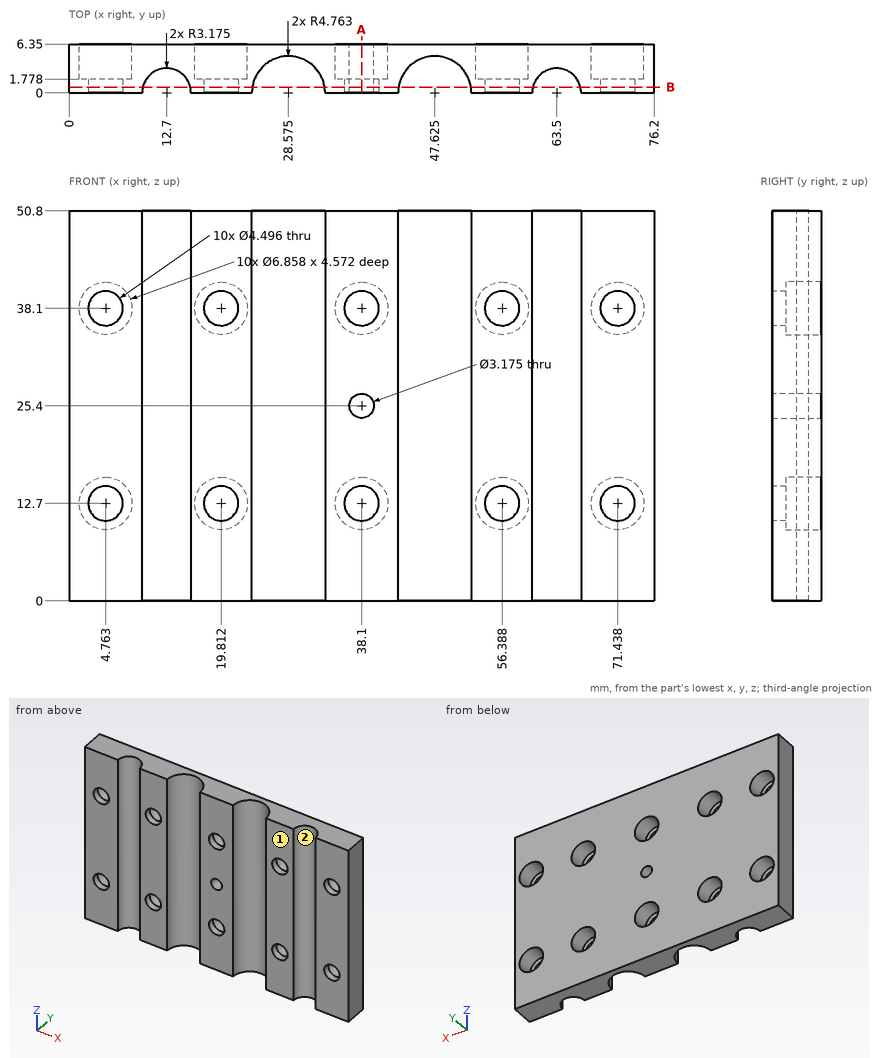
Check sheet for the drawn part. Datum: minimum x, y, z corner. Units: mm. Give positions to 0.01 mm unless a question says otherwise; leave off trailing zeros. Order: outer loops, then holes, each group sorted by start corner. A loop starts at its lowest first (then second) coordinate and runs counter-clockwise, first axis right, second up. Notation, with made-up numbers: (37.5, 43) -> (69.5, 43) arc R21 ccw to (69.5, 81) -> close; hole circle Ø7 at (13, 82.25). An arc over 180 degrees is marked (long way). One line per item, written item: value.
(1) Gauge pin test, flat end, axial feed: pin 1 (2 mm diameter, centred on x = 19.5, z = 14, fed in from +Y). Record the tip position at first contact, or that the pin passes through.
Final values:
pin 1: y = 1.78
(2) Scan lines: line 1 along Z through (x, y) = (35.5, 2) (1 decimal); line 2 along Z through (x, y) = (69.5, 2.5); line 3 along Z through (x, y) = (39, 0.5). Record each from-to range of solid material in increasing order. Write a range as [from, to].
Final values:
line 1: [0, 10.5], [14.9, 35.9], [40.3, 50.8]
line 2: [0, 9.87], [15.53, 35.27], [40.93, 50.8]
line 3: [0, 10.64], [14.76, 24.09], [26.71, 36.04], [40.16, 50.8]
(3) Sectioned sample at B-B on y = 0.75. Count the separate pieces of the cut face and the enclosed holes in it, then the cut area to 3 significant figures.
Final values:
separate pieces: 5
enclosed holes: 11
area: 2,120 mm^2
(4) Sectioned sample at A-A on x = 38.1. Record the cut outline in (y, z).
Final values:
outline: (0, 0) -> (6.35, 0) -> (6.35, 9.27) -> (1.78, 9.27) -> (1.78, 10.45) -> (0, 10.45) -> close; (0, 14.95) -> (1.78, 14.95) -> (1.78, 16.13) -> (6.35, 16.13) -> (6.35, 23.81) -> (0, 23.81) -> close; (0, 26.99) -> (6.35, 26.99) -> (6.35, 34.67) -> (1.78, 34.67) -> (1.78, 35.85) -> (0, 35.85) -> close; (0, 40.35) -> (1.78, 40.35) -> (1.78, 41.53) -> (6.35, 41.53) -> (6.35, 50.8) -> (0, 50.8) -> close
(5) Draft check along X on the marked faces 1 and 2. Enter one of: pulls with the +X half, pulls with the -X half, needs draft (parallel to the pull), parting line crosses it, or undercut.
Final values:
face 1: needs draft
face 2: undercut
